from build123d import *

# Parameters (mm, degrees)
F0_R     = 185
F1_DEPTH = 20
F4_R     = 2.5
F5_DEPTH = 5
F6_R     = 12.5
F7_DEPTH = 50


# Not quite as in the source:
# - the program builds the solid bodies; features that only make, move or delete a surface that nothing else refers to are left out


with BuildPart() as f1:
    # F0 (on Top) → F1 (new body)
    with BuildSketch(Plane.XY):
        Circle(F0_R)
    extrude(amount=F1_DEPTH)

    # F4 (on face) → F5 (cut)
    with BuildSketch(Plane.XY.offset(20)):
        Circle(F4_R)
        with Locations((0, 25)):
            Circle(F4_R)
        with Locations((0, 50)):
            Circle(F4_R)
        with Locations((0, 75)):
            Circle(F4_R)
        with Locations((0, 100)):
            Circle(F4_R)
        with Locations((0, 125)):
            Circle(F4_R)
        with Locations((25, 0)):
            Circle(F4_R)
        with Locations((25, 25)):
            Circle(F4_R)
        with Locations((25, 50)):
            Circle(F4_R)
        with Locations((25, 75)):
            Circle(F4_R)
        with Locations((25, 100)):
            Circle(F4_R)
        with Locations((25, 125)):
            Circle(F4_R)
        with Locations((50, 0)):
            Circle(F4_R)
        with Locations((50, 25)):
            Circle(F4_R)
        with Locations((50, 50)):
            Circle(F4_R)
        with Locations((50, 75)):
            Circle(F4_R)
        with Locations((50, 100)):
            Circle(F4_R)
        with Locations((50, 125)):
            Circle(F4_R)
        with Locations((75, 0)):
            Circle(F4_R)
        with Locations((75, 25)):
            Circle(F4_R)
        with Locations((75, 50)):
            Circle(F4_R)
        with Locations((75, 75)):
            Circle(F4_R)
        with Locations((75, 100)):
            Circle(F4_R)
        with Locations((75, 125)):
            Circle(F4_R)
        with Locations((100, 0)):
            Circle(F4_R)
        with Locations((100, 25)):
            Circle(F4_R)
        with Locations((100, 50)):
            Circle(F4_R)
        with Locations((100, 75)):
            Circle(F4_R)
        with Locations((100, 100)):
            Circle(F4_R)
        with Locations((125, 0)):
            Circle(F4_R)
        with Locations((125, 25)):
            Circle(F4_R)
        with Locations((125, 50)):
            Circle(F4_R)
        with Locations((125, 75)):
            Circle(F4_R)
        with Locations((75, -25)):
            Circle(F4_R)
        with Locations((100, -50)):
            Circle(F4_R)
        with Locations((0, -100)):
            Circle(F4_R)
        with Locations((100, -100)):
            Circle(F4_R)
        with Locations((75, -100)):
            Circle(F4_R)
        with Locations((125, -50)):
            Circle(F4_R)
        with Locations((75, -125)):
            Circle(F4_R)
        with Locations((25, -50)):
            Circle(F4_R)
        with Locations((0, -75)):
            Circle(F4_R)
        with Locations((100, -75)):
            Circle(F4_R)
        with Locations((100, -25)):
            Circle(F4_R)
        with Locations((50, -125)):
            Circle(F4_R)
        with Locations((125, -25)):
            Circle(F4_R)
        with Locations((50, -75)):
            Circle(F4_R)
        with Locations((25, -25)):
            Circle(F4_R)
        with Locations((75, -75)):
            Circle(F4_R)
        with Locations((75, -50)):
            Circle(F4_R)
        with Locations((125, -75)):
            Circle(F4_R)
        with Locations((0, -125)):
            Circle(F4_R)
        with Locations((25, -75)):
            Circle(F4_R)
        with Locations((50, -100)):
            Circle(F4_R)
        with Locations((25, -125)):
            Circle(F4_R)
        with Locations((0, -50)):
            Circle(F4_R)
        with Locations((25, -100)):
            Circle(F4_R)
        with Locations((50, -25)):
            Circle(F4_R)
        with Locations((50, -50)):
            Circle(F4_R)
        with Locations((0, -25)):
            Circle(F4_R)
        with Locations((-25, -75)):
            Circle(F4_R)
        with Locations((-50, -100)):
            Circle(F4_R)
        with Locations((-100, 0)):
            Circle(F4_R)
        with Locations((-100, -100)):
            Circle(F4_R)
        with Locations((-100, -75)):
            Circle(F4_R)
        with Locations((-50, -125)):
            Circle(F4_R)
        with Locations((-125, -75)):
            Circle(F4_R)
        with Locations((-50, -25)):
            Circle(F4_R)
        with Locations((-75, 0)):
            Circle(F4_R)
        with Locations((-75, -100)):
            Circle(F4_R)
        with Locations((-25, -100)):
            Circle(F4_R)
        with Locations((-125, -50)):
            Circle(F4_R)
        with Locations((-25, -125)):
            Circle(F4_R)
        with Locations((-75, -50)):
            Circle(F4_R)
        with Locations((-25, -25)):
            Circle(F4_R)
        with Locations((-75, -75)):
            Circle(F4_R)
        with Locations((-50, -75)):
            Circle(F4_R)
        with Locations((-75, -125)):
            Circle(F4_R)
        with Locations((-125, 0)):
            Circle(F4_R)
        with Locations((-75, -25)):
            Circle(F4_R)
        with Locations((-100, -50)):
            Circle(F4_R)
        with Locations((-125, -25)):
            Circle(F4_R)
        with Locations((-50, 0)):
            Circle(F4_R)
        with Locations((-100, -25)):
            Circle(F4_R)
        with Locations((-25, -50)):
            Circle(F4_R)
        with Locations((-50, -50)):
            Circle(F4_R)
        with Locations((-25, 0)):
            Circle(F4_R)
        with Locations((-75, 25)):
            Circle(F4_R)
        with Locations((-100, 50)):
            Circle(F4_R)
        with Locations((-100, 100)):
            Circle(F4_R)
        with Locations((-75, 100)):
            Circle(F4_R)
        with Locations((-125, 50)):
            Circle(F4_R)
        with Locations((-75, 125)):
            Circle(F4_R)
        with Locations((-25, 50)):
            Circle(F4_R)
        with Locations((-100, 75)):
            Circle(F4_R)
        with Locations((-100, 25)):
            Circle(F4_R)
        with Locations((-50, 125)):
            Circle(F4_R)
        with Locations((-125, 25)):
            Circle(F4_R)
        with Locations((-50, 75)):
            Circle(F4_R)
        with Locations((-25, 25)):
            Circle(F4_R)
        with Locations((-75, 75)):
            Circle(F4_R)
        with Locations((-75, 50)):
            Circle(F4_R)
        with Locations((-125, 75)):
            Circle(F4_R)
        with Locations((-25, 75)):
            Circle(F4_R)
        with Locations((-50, 100)):
            Circle(F4_R)
        with Locations((-25, 125)):
            Circle(F4_R)
        with Locations((-25, 100)):
            Circle(F4_R)
        with Locations((-50, 25)):
            Circle(F4_R)
        with Locations((-50, 50)):
            Circle(F4_R)
    extrude(amount=-F5_DEPTH, mode=Mode.SUBTRACT)

    # F6 (on face) → F7 (join)
    with BuildSketch(Plane.XY.offset(20)):
        with Locations((-135.6773132596, 0)):
            Circle(F6_R)
        with Locations((67.8386566298, -117.5)):
            Circle(F6_R)
        with Locations((67.8386566298, 117.5)):
            Circle(F6_R)
    extrude(amount=F7_DEPTH)


solid = f1.part
Can you work these out from the model? Positions are in its coordinate system, mm. A direction names the side the tool comes from. Give positions to 0.01 mm unless a question says otherwise; leave off trailing zeros. Write each loop counter-clockwise with the first axis right and the second up, starting at its lowest first coordinate (ties: lowest second). Pieces come first, ordered by that corner, then holes. Notation, with made-up numbers: (54.5, 53.25) -> (97.5, 53.25) arc R7 ccw to (97.5, 61.25) -> close; hole circle Ø5 at (-30, 17.25). An arc over 180 degrees is marked (long way). Answer as a JSON object with one key per item and string values. Group by question number.
Item 1: Suppose I cut it at C-C (y = -117.5). Please give me the cut outline in (x, z), plus the area to 3 significant figures.
Item 2: Suppose I cut it at A-A (x = -142). Please give me the cut outline in (y, z), plus the area to 3 significant figures.
Item 3: Please list where these lines run through material, in increasing order: line 1 (Z direction, x = -32, y = -161); line 2 (Y direction, x = 60, z = 65); line 3 (X direction, y = 95, z = 4). Write a range as [from, to].
Item 4: We'd pull the mould along Y, two halves only. Please class faces 1 (the face through (74.56, -106.96, 44.65)), 2 (the face through (-136, 0, 70)), 3 (the face through (-123.755, 3.755, 44.65)): +Y half, -Y half, draft (parallel to the pull), parting line (faces both ways), or undercut.
Item 5: For faces 4 (the face through (68, 118, 70)), 5 (the face through (74.56, 128.04, 44.65)), which set-ups out of +Z, -Z, +X, -X, +Y, -Y let a thin tool reach every point of the face, with its end or its side?
Item 6: Suppose I cut it at B-B (z = 34). Please give me the cut outline in (x, y), plus the area to 3 significant figures.
Item 7: I'm going to push flat-ended pins straight in: P1, Ø5.5, axis at x = 0, y = -50.5, coming from the +Z side; P2, Ø2.5, axis at x = 26, y = 50.5, coming from the +Z side; P3, Ø5, axis at x = -118, z = 11, coming from the -Y side. Where does each tip first touch, or does it pass through?
Item 8: Suppose I cut it at D-D (z = 8). Please give me the cut outline in (x, y).
Findings:
{
 "1": {"outline": "(-142.89, 0) -> (142.89, 0) -> (142.89, 20) -> (80.34, 20) -> (80.34, 70) -> (55.34, 70) -> (55.34, 20) -> (-142.89, 20) -> close", "area": "6,970 mm²"},
 "2": {"outline": "(-118.58, 0) -> (118.58, 0) -> (118.58, 20) -> (10.78, 20) -> (10.78, 70) -> (-10.78, 70) -> (-10.78, 20) -> (-118.58, 20) -> close", "area": "5,820 mm²"},
 "3": {"line 1": "z = [0, 20]", "line 2": "y = [-127.24, -107.76], [107.76, 127.24]", "line 3": "x = [-158.75, 158.75]"},
 "4": {"face 1": "undercut", "face 2": "draft", "face 3": "parting line"},
 "5": {"face 4": "+Z, +X, -X, +Y, -Y", "face 5": "+Z"},
 "6": {"outline": "circle Ø25 at (-135.68, 0); circle Ø25 at (67.84, -117.5); circle Ø25 at (67.84, 117.5)", "area": "1,470 mm²"},
 "7": {"P1": "stops at z = 20", "P2": "stops at z = 15", "P3": "stops at y = -144.52"},
 "8": {"outline": "circle Ø370 at (0, 0)"}
}
